Here's how the part is built. I have some questions about the finished solid (model axes, mm). A direction names the side the tool comes from. Coordinates: 2 decimals unless noted, no trailing zeros. Loops run counter-clockwise (first coordinate to the right, second up) from the corner with the lowest first, then second, coordinate; pieces in that order, holes last. Notation, with made-up numbers: (89.5, 18.25) - (147.5, 18.25) arc R28 cw to (147.5, 52.25) - close; hole circle Ø3 at (12.25, 44). An arc over 180 degrees is marked (long way). Use a Markdown table: item, result.
```python
from build123d import *

# Parameters (mm, degrees)
F0_W     = 24
F0_H     = 74
F0_W_2   = 20
F0_H_2   = 70
F1_DEPTH = 25
F2_R     = 2
F3_R     = 1.99999


# Not quite as in the source:
# - a fillet or chamfer is up to 0.001 mm smaller than in the source, because OpenCascade refuses the exact size


with BuildPart() as f1:
    # F0 (on Top) → F1 (new body)
    with BuildSketch(Plane.XY):
        Rectangle(F0_W, F0_H)
        Rectangle(F0_W_2, F0_H_2, mode=Mode.SUBTRACT)
    extrude(amount=F1_DEPTH)

    # F2
    f2_edges = [f1.edges().sort_by_distance(p)[0] for p in [
        (-12, -37, 12.5),
        (12, -37, 12.5),
        (12, 37, 12.5),
        (-12, 37, 12.5),
    ]]
    fillet(f2_edges, radius=F2_R)

    # F3 (radius 2 in the source; OpenCascade refuses exactly that, so slightly less here)
    f3_edges = [f1.edges().sort_by_distance(p)[0] for p in [
        (-12, 0, 25),
    ]]
    fillet(f3_edges, radius=F3_R)


solid = f1.part
```
Q1. I want a section at C-C, the plane z = 20.5. Write out the boundary of the cut face in (x, y), then the cut area to 3 significant figures.
Check values:
| item | result |
|---|---|
| outline | (-12, -35) arc R2 ccw to (-10, -37) - (10, -37) arc R2 ccw to (12, -35) - (12, 35) arc R2 ccw to (10, 37) - (-10, 37) arc R2 ccw to (-12, 35) - close; hole (-10, -35) - (10, -35) - (10, 35) - (-10, 35) - close |
| area | 373 mm^2 |
Q2. Please list where these lines run through material, in increasing order: L1, parallel to Y at x = 9.25, z = 18; L2, parallel to X at y = 28, z = 9.25; L3, parallel to Y at x = -10.25, z = 12.5. Write a range as from..to.
Check values:
| item | result |
|---|---|
| L1 | -37..-35, 35..37 |
| L2 | -12..-10, 10..12 |
| L3 | -36.98..36.98 |
Q3. Which directions (+Z, -Z, +X, -X, +Y, -Y) give clear straight access to the entire face, cutting with the end or side of a thin tool? Please do faces 5 (the face through (-10, 0, 12)), 6 (the face through (0, 37, 11)).
Check values:
| item | result |
|---|---|
| face 5 | +Z, -Z |
| face 6 | +Z, -Z, +X, -X, +Y |
Q4. If we mould it in two halves opening along Y, with no side actions, what happens to faces 1 (the face through (10, 0, 12)), 2 (the face through (11.4, 36.43, 11.66)), 3 (the face through (-11.43, -36.4, 11.66)), 4 (the face through (11.43, -0.49, 24.4))? For each: pulls with the +Y half, pulls with the -Y half, needs draft (parallel to the pull), parting line crosses it, or undercut.
Check values:
| item | result |
|---|---|
| face 1 | undercut |
| face 2 | pulls with the +Y half |
| face 3 | pulls with the -Y half |
| face 4 | needs draft |
